Source: CAD feature listing. Evaluate the final solid. Frame: model axes, mm. A direction names the side the tool comes from. Give positions to 0.01 mm unless a question says otherwise; leave off trailing zeros. Loops run counter-clockwise (first coordinate to the right, second up) from the corner with the lowest first, then second, coordinate; pieces in that order, holes last.
from build123d import *

# Parameters (mm, degrees)
F1_DEPTH = 83
F0_W     = 37
F0_H     = 2.4
F2_DEPTH = 38
F3_DEPTH = 3
F4_D     = 4
F5_D     = 4
F7_DEPTH = 2
F8_DEPTH = 2
F10_D    = 2


with BuildPart() as f1:
    # F0 (on Front) → F1 (new body)
    with BuildSketch(Plane.XZ):
        with BuildLine():
            Line((-65, 6.656936314), (0, 6.656936314))
            Line((0, 6.656936314), (0, 9.456936314))
            Line((0, 9.456936314), (-65, 9.456936314))
            ThreePointArc((-65, 9.456936314), (-65.3535533906, 9.3104897046), (-65.5, 8.956936314))
            Line((-65.5, 8.956936314), (-65.5, 7.156936314))
            ThreePointArc((-65.5, 7.156936314), (-65.3535533906, 6.8033829234), (-65, 6.656936314))
        make_face()
        with BuildLine():
            Line((0, 9.456936314), (0, 6.656936314))
            Line((0, 6.656936314), (65, 6.656936314))
            ThreePointArc((65, 6.656936314), (65.3535533906, 6.8033829234), (65.5, 7.156936314))
            Line((65.5, 7.156936314), (65.5, 8.956936314))
            ThreePointArc((65.5, 8.956936314), (65.3535533906, 9.3104897046), (65, 9.456936314))
            Line((65, 9.456936314), (0, 9.456936314))
        make_face()
    extrude(amount=F1_DEPTH)



with BuildPart() as f2:
    # F0 (on Front) → F2 (new body)
    with BuildSketch(Plane.XZ):
        with Locations((-18.5, 16.156936314)):
            Rectangle(F0_W, F0_H)
        with Locations((18.5, 16.156936314)):
            Rectangle(F0_W, F0_H)
    extrude(amount=F2_DEPTH)


with BuildPart() as f1_1:
    add(f1.part)

    add(f2.part)  # F3 merges F2
    # F0 (on Front) → F3 (join)
    with BuildSketch(Plane.XZ):
        with BuildLine():
            ThreePointArc((-50.9090917143, 71.1945314942), (-60.4545458571, 79.1209226904), (-70, 71.1945314942))
            Line((-70, 71.1945314942), (-50.9090917143, 71.1945314942))
        make_face()
        with BuildLine():
            Line((50.9090917143, 71.1945314942), (70, 71.1945314942))
            ThreePointArc((70, 71.1945314942), (60.4545458571, 79.1209226904), (50.9090917143, 71.1945314942))
        make_face()
        with BuildLine():
            Line((0, 6.656936314), (0, 0))
            Line((0, 0), (67, 0))
            ThreePointArc((67, 0), (69.1213203436, 0.8786796564), (70, 3))
            Line((70, 3), (70, 71.1945314942))
            Line((70, 71.1945314942), (50.9090917143, 71.1945314942))
            Line((50.9090917143, 71.1945314942), (42.8696187161, 28.1887182873))
            ThreePointArc((42.8696187161, 28.1887182873), (41.8372358629, 26.4319780432), (39.9207030491, 25.7399862697))
            Line((39.9207030491, 25.7399862697), (0, 25.7399862697))
            Line((0, 25.7399862697), (0, 17.356936314))
            Line((0, 17.356936314), (37, 17.356936314))
            Line((37, 17.356936314), (37, 14.956936314))
            Line((37, 14.956936314), (0, 14.956936314))
            Line((0, 14.956936314), (0, 9.456936314))
            Line((0, 9.456936314), (65, 9.456936314))
            ThreePointArc((65, 9.456936314), (65.3535533906, 9.3104897046), (65.5, 8.956936314))
            Line((65.5, 8.956936314), (65.5, 7.156936314))
            ThreePointArc((65.5, 7.156936314), (65.3535533906, 6.8033829234), (65, 6.656936314))
            Line((65, 6.656936314), (0, 6.656936314))
        make_face()
        with BuildLine():
            Line((-70, 71.1945314942), (-70, 3))
            ThreePointArc((-70, 3), (-69.1213203436, 0.8786796564), (-67, 0))
            Line((-67, 0), (0, 0))
            Line((0, 0), (0, 6.656936314))
            Line((0, 6.656936314), (-65, 6.656936314))
            ThreePointArc((-65, 6.656936314), (-65.3535533906, 6.8033829234), (-65.5, 7.156936314))
            Line((-65.5, 7.156936314), (-65.5, 8.956936314))
            ThreePointArc((-65.5, 8.956936314), (-65.3535533906, 9.3104897046), (-65, 9.456936314))
            Line((-65, 9.456936314), (0, 9.456936314))
            Line((0, 9.456936314), (0, 14.956936314))
            Line((0, 14.956936314), (-37, 14.956936314))
            Line((-37, 14.956936314), (-37, 17.356936314))
            Line((-37, 17.356936314), (0, 17.356936314))
            Line((0, 17.356936314), (0, 25.7399862697))
            Line((0, 25.7399862697), (-39.9207030491, 25.7399862697))
            ThreePointArc((-39.9207030491, 25.7399862697), (-41.8372358629, 26.4319780432), (-42.8696187161, 28.1887182873))
            Line((-42.8696187161, 28.1887182873), (-50.9090917143, 71.1945314942))
            Line((-50.9090917143, 71.1945314942), (-70, 71.1945314942))
        make_face()
    extrude(amount=F3_DEPTH)

    # F4 (through all)
    with Locations(Plane(origin=(0, 0, 0), x_dir=(1, 0, 0), z_dir=(0, 1, 0))):
        with Locations((-60.4545458571, -69.4101117817)):
            Hole(F4_D / 2)

    # F5 (through all)
    with Locations(Plane(origin=(0, 0, 0), x_dir=(1, 0, 0), z_dir=(0, 1, 0))):
        with Locations((60.4545458571, -69.4101117817)):
            Hole(F5_D / 2)

    # F6 (on Right) → F7 (join, symmetric)
    with BuildSketch(Plane.YZ):
        Polygon((-53.0555397272, 6.8902592175), (0, 0), (0, 6.8902592175), align=None)
    extrude(amount=F7_DEPTH, both=True)

    # F6 (on Right) → F8 (join, symmetric)
    with BuildSketch(Plane.YZ):
        Polygon((-30.1237229723, 17.327228561), (-2.9568942264, 17.3339545727), (-2.9568942264, 21.6480610112), align=None)
    extrude(amount=F8_DEPTH, both=True)

    # F10 (through all)
    with Locations(Plane.XY.offset(17.356936314)):
        with Locations((32, -33)):
            Hole(F10_D / 2)


solid = f1_1.part
1) Cut plane C-C (x = -28). Return loops of the section in (y, z).
Checks:
outline: (-83, 6.66) - (-3, 6.66) - (-3, 0) - (0, 0) - (0, 25.74) - (-3, 25.74) - (-3, 17.36) - (-38, 17.36) - (-38, 14.96) - (-3, 14.96) - (-3, 9.46) - (-83, 9.46) - close
2) Cut plane B-B (y = -12). Return loops of the section in (x, z).
Checks:
outline: (-65.5, 7.16) arc R0.5 ccw to (-65, 6.66) - (-2, 6.66) - (-2, 1.56) - (2, 1.56) - (2, 6.66) - (65, 6.66) arc R0.5 ccw to (65.5, 7.16) - (65.5, 8.96) arc R0.5 ccw to (65, 9.46) - (-65, 9.46) arc R0.5 ccw to (-65.5, 8.96) - close; (-37, 14.96) - (37, 14.96) - (37, 17.36) - (2, 17.36) - (2, 20.21) - (-2, 20.21) - (-2, 17.36) - (-37, 17.36) - close
3) Reachability of faces 1 (the flat face through (2, -17, 5)), 2 (the flat face through (46.946, -1.479, 49.993)), 3 (the flat face through (1, -42, 9.457)), 4 (the flat face through (-2, -17, 5)), 5 (the flat face through (2, -11, 19)) from +Z, -Z, +X, -X, +Y, -Y: full face, straight path, thin tool, end or side. Return the list, or none.
Checks:
face 1: -Z, +X, -Y
face 2: +Z, +Y, -Y
face 3: +X, -X, -Y
face 4: -Z, -X, -Y
face 5: +Z, +X, -Y
4) Cut plane D-D (z = 33.5). Return loops of the section in (x, y), and give its area (3 significant figures).
Checks:
outline: (-70, -3) - (-43.86, -3) - (-43.86, 0) - (-70, 0) - close; (43.86, -3) - (70, -3) - (70, 0) - (43.86, 0) - close
area: 157 mm2
5) Contact query for flat-ended pins moving along their axis: P1, Ø0.7, axis at y = -22.5, z = 16.5, coming from the -X side; P2, Ø24, axis at x = -31, y = -35.5, coming from the -Z side; P3, Ø2.5, axis at y = -27, z = 16, coming from the +X side. Output: stop coordinate, or through.
Checks:
P1: stops at x = -37
P2: stops at z = 6.66
P3: stops at x = 37
6) Cut plane A-A (z = 51). Return loops of the section in (x, y), and give its area (3 significant figures).
Checks:
outline: (-70, -3) - (-47.13, -3) - (-47.13, 0) - (-70, 0) - close; (47.13, -3) - (70, -3) - (70, 0) - (47.13, 0) - close
area: 137 mm2
7) Pull-direction query (X, two-part tool) for faces 6 (the cylindrical face through (69.1, -1.48, 0.86)), 7 (the flat face through (-1, -1, 0)), 8 (the flat face through (1, -1, 25.74)); classes: released by +X, released by -X, zero draft, split by the parting line, or undercut.
Checks:
face 6: released by +X
face 7: zero draft
face 8: undercut
8) Ray query, probe 1 along Y at (x, z) = (32, 7.7); probe 2 along Z at (x, y) = (-19.5, -13.5); probe 3 along Z at (x, y) = (-11, -46.5). Return the intervals inside material, ascending.
Checks:
probe 1: y = -83 to -34, -32 to 0
probe 2: z = 6.66 to 9.46, 14.96 to 17.36
probe 3: z = 6.66 to 9.46
